```python
from build123d import *

# Parameters (mm, degrees)
F1_DEPTH = 63.5
F2_R     = 27.3812
F3_DEPTH = 101.6


# Not quite as in the source:
# - a feature names something its author has since deleted; it is built from what else it names


with BuildPart() as f1:
    # F0 (on Front) → F1 (new body)
    with BuildSketch(Plane.XZ):
        with BuildLine():
            ThreePointArc((-3.7017028225, 34.7282740892), (1.3544064685, 34.8987278868), (6.3820971775, 34.3369256139))
            Line((6.3820971775, 34.3369256139), (6.3820971775, 57.1461256139))
            Line((6.3820971775, 57.1461256139), (-3.7017028225, 57.1461256139))
            Line((-3.7017028225, 57.1461256139), (-3.7017028225, 34.7282740892))
        make_face()
        with BuildLine():
            Line((5.6386164435, -49.9173291028), (5.6386164435, -34.4668192557))
            ThreePointArc((5.6386164435, -34.4668192557), (0.6030353105, -34.9197934332), (-4.4451835565, -34.6409579566))
            Line((-4.4451835565, -34.6409579566), (-4.4451835565, -49.9173291028))
            Line((-4.4451835565, -49.9173291028), (5.6386164435, -49.9173291028))
        make_face()
        with BuildLine():
            ThreePointArc((5.6386164435, -34.4668192557), (26.6146980472, -22.6144527428), (34.925, 0))
            ThreePointArc((34.925, 0), (26.8574977327, 22.3255557722), (6.3820971775, 34.3369256139))
            ThreePointArc((6.3820971775, 34.3369256139), (1.3544064685, 34.8987278868), (-3.7017028225, 34.7282740892))
            ThreePointArc((-3.7017028225, 34.7282740892), (-34.9229942598, 0.3742952407), (-4.4451835565, -34.6409579566))
            ThreePointArc((-4.4451835565, -34.6409579566), (0.6030353105, -34.9197934332), (5.6386164435, -34.4668192557))
        make_face()
    extrude(amount=F1_DEPTH)

    # F2 (on face) → F3 (cut)
    with BuildSketch(Plane.XZ.offset(63.5)):
        Circle(F2_R)
    extrude(amount=-F3_DEPTH, mode=Mode.SUBTRACT)


solid = f1.part
```
Could you check a few things on this model? Use its own coordinates, in mm. A direction names the side the tool comes from. Round coordinates to 2 decimals unless told otherwise and drop trailing zeros. Write each loop counter-clockwise with the first axis right and the second up, starting at its lowest first coordinate (ties: lowest second). Pieces come first, ordered by that corner, then holes. Notation, with made-up numbers: M 20,-15 L 38,-15 A22 ccw 38,11 Z; hole C 62.5,-19 d9. An arc over 180 degrees is marked long. Answer in a Markdown table with one row per item. Add a question column.
Q1. Will these pins go through, and if not, where does the flat tip stop? pin 1 Ø6.5 at (y, z) = (-25, 42) entering from -X; pin 2 Ø7.5 at (y, z) = (-21, -45.5) entering from -X; pin 3 Ø4.5 at (y, z) = (-17.5, -40) entering from +X; pin 4 Ø5 at (x, z) = (-9.5, 37.5) entering from +Y.
Q2. On a 3-axis mill with a long thin cutter (end or side, diameter ignored), from which of +Z, -Z, +X, -X, +Y, -Y can I reach the whole of each face in a straight line? I mean faces 4 (the flat face through (-3, -63.5, 28)), 5 (the flat face through (5.639, -31, -42)), 6 (the flat face through (-3, 0, 28)), 7 (the flat face through (-3.702, -31, 46)), 8 (the flat face through (-4.445, -31, -42)). Say none if no direction works.
Q3. Imagine slicing it at B-B (z = 0). Please give me the cut outline in (x, y) (3 decimals).
Q4. Imagine slicing it at D-D (z = 41). Please give me the cut outline in (x, y), then the cut area to 3 significant figures.
Q5. If I drill on line 1 (Z direction, x = 0, y = -36); line 2 (Z direction, x = 22, y = -49); line 3 (X direction, y = -17, z = -17), over which ranges is the centre line in solid material (lowest first)? Write a range as from..to.
Q6. Imagine slicing it at A-A (x = 0). Please give me the cut outline in (y, z), then the cut area to 3 significant figures.
Q7. Imagine slicing it at C-C (y = -38). Please give me the cut outline in (x, z) (3 decimals).
Q8. If we mould it in two halves opening along Z, with no side actions, what happens to faces 1 (the cylindrical face through (-3.56, -32.19, 27.15)), 2 (the flat face through (1, -31, 57.146)), 3 (the flat face through (6.382, -31, 46))? For each: +Z half, -Z half, draft (parallel to the pull), parting line (faces both ways), or undercut.
Values:
| question | item | result |
|---|---|---|
| 1 | pin 1 | x = -3.7 |
| 1 | pin 2 | x = -4.45 |
| 1 | pin 3 | x = 5.64 |
| 1 | pin 4 | through |
| 2 | face 4 | +Z, -Z, +X, -X, -Y |
| 2 | face 5 | -Z, +X, +Y, -Y |
| 2 | face 6 | +Z, -Z, +X, -X, +Y |
| 2 | face 7 | +Z, -X, +Y, -Y |
| 2 | face 8 | -Z, -X, +Y, -Y |
| 3 | outline | M -34.925,-63.5 L -27.381,-63.5 L -27.381,0 L -34.925,0 Z; M 27.381,-63.5 L 34.925,-63.5 L 34.925,0 L 27.381,0 Z |
| 4 | outline | M -3.7,-63.5 L 6.38,-63.5 L 6.38,0 L -3.7,0 Z |
| 4 | area | 640 mm^2 |
| 5 | line 1 | -49.92..-27.38, 27.38..57.15 |
| 5 | line 2 | -27.12..-16.3, 16.3..27.12 |
| 5 | line 3 | -30.51..-21.46, 21.46..30.51 |
| 6 | outline | M -63.5,-49.92 L 0,-49.92 L 0,-27.38 L -63.5,-27.38 Z; M -63.5,27.38 L 0,27.38 L 0,57.15 L -63.5,57.15 Z |
| 6 | area | 3,320 mm^2 |
| 7 | outline | M -4.445,-49.917 L 5.639,-49.917 L 5.639,-34.467 A34.925 ccw 6.382,34.337 L 6.382,57.146 L -3.702,57.146 L -3.702,34.728 A34.925 ccw -4.445,-34.641 Z; hole C 0,0 d54.762 |
| 8 | face 1 | undercut |
| 8 | face 2 | +Z half |
| 8 | face 3 | draft |
